The model under review builds one solid part; all positions refer to its coordinate system, in mm. A direction names the side the tool comes from. Give positions to 0.01 mm unless a question says otherwise; leave off trailing zeros. Loops run counter-clockwise (first coordinate to the right, second up) from the corner with the lowest first, then second, coordinate; pieces in that order, holes last. Notation, with made-up numbers: (42, -23.5) - (69, -23.5) arc R15 ccw to (69, 3.5) - close; hole circle Ø6 at (-18.75, 71.5). An arc over 180 degrees is marked (long way). Answer as a JSON object with one key per item and string values.
Autodesk Inventor part; units mm, degrees
ref_plane "YZ Plane" through (0, 0, 0) normal (1, 0, 0) x (0, 1, 0)
ref_plane "XZ Plane" through (0, 0, 0) normal (0, 1, 0) x (-1, 0, 0)
ref_plane "XY Plane" through (0, 0, 0) normal (0, 0, 1) x (1, 0, 0)
sketch "Sketch1" plane through (0, 0, 0) normal (0, 1, 0) x (-1, 0, 0)
  line L0 (-6, 8.5) -> (6, 8.5)
  line L1 (6, 8.5) -> (6, -8.5)
  line L2 (6, -8.5) -> (-6, -8.5)
  line L3 (-6, -8.5) -> (-6, 8.5)
  line L4 (-6, 8.5) -> (6, -8.5) construction
  line L5 (6, 8.5) -> (-6, -8.5) construction
  point P0 (0, 0)
  dimension "d0" = 12
  dimension "d1" = 17
extrude "Extrusion1" add sketch "Sketch1" along normal blind 0.5
sketch "Sketch2" plane through (0, 0.5, 0) normal (0, 1, 0) x (1, 0, 0)
  line L0 (5.1, -7.6) -> (-5.1, -7.6)
  line L1 (-5.1, -7.6) -> (-5.1, 7.6)
  line L2 (-5.1, 7.6) -> (5.1, 7.6)
  line L3 (5.1, 7.6) -> (5.1, -7.6)
  line L4 (5.1, -7.6) -> (-5.1, 7.6) construction
  line L5 (-5.1, -7.6) -> (5.1, 7.6) construction
  point P0 (0, 0)
  dimension "d4" = 15.2
  dimension "d5" = 10.2
extrude "Extrusion2" add sketch "Sketch2" along normal blind 0.75
fillet "Fillet1" radius 1.5 4 edges at (-6, 0.25, 8.5) (6, 0.25, 8.5) (6, 0.25, -8.5) (-6, 0.25, -8.5)
fillet "Fillet2" radius 0.5 4 edges at (5.1, 0.875, -7.6) (-5.1, 0.875, -7.6) (-5.1, 0.875, 7.6) (5.1, 0.875, 7.6)
sketch "Sketch3" plane through (0, 0, 0) normal (0, -1, 0) x (1, 0, 0)
  line L0 (5, 0) -> (3.5, 0)
  line L1 (2.5, -1) -> (2.5, -5.5)
  line L2 (3.5, -6.5) -> (5, -6.5)
  line L3 (5, -6.5) -> (5, 0)
  line L4 (5, 0) -> (8.5853, 0)
  line L5 (8.5853, 0) -> (8.5853, -6.5)
  line L6 (8.5853, -6.5) -> (5, -6.5)
  line L7 (5, -6.5) -> (5, 0)
  line L8 (4.5, -8.5) -> (-4.5, -8.5)
  line L9 (6, 7) -> (6, -7)
  circle A0 centre (0, -4) radius 1
  line L10 (-6, -7) -> (-6, 7)
  arc A1 (3.5, 0) -> (2.5, -1) centre (3.5, -1) ccw
  arc A2 (2.5, -5.5) -> (3.5, -6.5) centre (3.5, -5.5) ccw
  point P0 (0, 0)
  point P1 (2.5, -6.5)
  point P2 (6, -6.5)
  point P3 (6, 0)
  dimension "d10" = 6.5
  dimension "d11" = 2.5
  dimension "d12" = 2
  dimension "d13" = 3.5
  dimension "d14" = 6
  dimension "d15" = 4.5
  dimension "d16" = 2
  dimension "d17" = 1
extrude "Extrusion3" cut sketch "Sketch3" against normal up to surface (1.25 mm away) contours L3 L2 A2 L1 A1 L0 | L4 L9 L6 L3 | A0
fillet "Fillet3" radius 0.5 4 edges at (5.1, 0.875, 0) (5.1, 0.875, -6.5) (6, 0.25, -6.5) (6, 0.25, 0)
properties part number "proxima_cup"
Q1. The part is to be moulded in two halves that separate along X. For faces 1 (the face through (-5.57, 0.25, 8.05)), 2 (the face through (5.57, 0.25, -8.05)), 3 (the face through (0, 1, -3)), 4 (the face through (0, 1.25, 0)), say which applies: +X half, -X half, draft (parallel to the pull), parting line (faces both ways), or undercut.
Results:
{"face 1": "-X half", "face 2": "+X half", "face 3": "undercut", "face 4": "draft"}
Q2. Clearance check with a flat-ended pin moving along its axis: pin 1 Ø0.6 at (y, z) = (0.5, -2.5) entering from +X. State where the tip first meets the part, or that it passes through.
Results:
{"pin 1": "stops at x = 2.5"}
Q3. To check wall thickness, follow probe 1 along Z at (x, y) = (0, 0.55); probe 2 along Z at (x, y) = (4, 0.6); probe 3 along X at (y, z) = (1, 2.75). State the ranges of each line that lie inside material, in increasing order. Write a range as [from, to].
Results:
{"probe 1": "z = [-7.6, -5], [-3, 7.6]", "probe 2": "z = [-7.6, -6.5], [0, 7.6]", "probe 3": "x = [-5.1, 5.1]"}
Q4. For faces 5 (the face through (4.3, 0.5, 0)), 6 (the face through (0, 0, 0)), 7 (the face through (-5.3, 0.5, 0)), list the 3-axis set-ups (+Z, -Z, +X, -X, +Y, -Y) from which the entire face can be reached by the end or side of a thin tool; tool diameter is ignored.
Results:
{"face 5": "+X, +Y, -Y", "face 6": "+Z, -Z, +X, -X, -Y", "face 7": "+Y"}
Q5. Consider section D-D, the plane z = 6.25. State the section outline as (x, y) points, plus the area to 4 significant figures.
Results:
{"outline": "(-6, 0) - (6, 0) - (6, 0.5) - (5.1, 0.5) - (5.1, 1.25) - (-5.1, 1.25) - (-5.1, 0.5) - (-6, 0.5) - close", "area": "13.65 mm^2"}
Q6. Consider section A-A, the plane z = -4. State the section outline as (x, y) points, plus the area to 3 significant figures.
Results:
{"outline": "(-6, 0) - (-1, 0) - (-1, 1.25) - (-5.1, 1.25) - (-5.1, 0.5) - (-6, 0.5) - close; (1, 0) - (2.5, 0) - (2.5, 1.25) - (1, 1.25) - close", "area": "7.45 mm^2"}
Q7. Consider section B-B, the plane x = 0. State the section outline as (y, z) points.
Results:
{"outline": "(0, -8.5) - (0.5, -8.5) - (0.5, -7.6) - (1.25, -7.6) - (1.25, -5) - (0, -5) - close; (0, -3) - (1.25, -3) - (1.25, 7.6) - (0.5, 7.6) - (0.5, 8.5) - (0, 8.5) - close"}
